Geometry check sheet. Reference: the model listing, model coordinates, mm. A direction names the side the tool comes from. Round coordinates to 2 decimals unless told otherwise and drop trailing zeros. Write each loop counter-clockwise with the first axis right and the second up, starting at its lowest first coordinate (ties: lowest second). Pieces come first, ordered by that corner, then holes. Notation, with made-up numbers: (27.5, 21.5) -> (84.5, 21.5) arc R24 ccw to (84.5, 57.5) -> close; hole circle Ø2 at (86, 55). An arc over 180 degrees is marked (long way). One line per question, with ' | ' between items.
```python
from build123d import *

# Parameters (mm, degrees)
ESQUISSE1_W                = 50
ESQUISSE1_H                = 10
BOSS_EXTRU_1_DEPTH         = 100
ESQUISSE2_R                = 5
BOSS_EXTRU_2_DEPTH         = 15
ESQUISSE3_R                = 5
BOSS_EXTRU_3_DEPTH         = 15
ESQUISSE4_W                = 10
ESQUISSE4_H                = 10
ENL_V_MAT_EXTRU_1_DEPTH    = 15
R_P_TITION_LIN_AIRE1_COUNT = 5
R_P_TITION_LIN_AIRE1_PITCH = 20
ESQUISSE5_W                = 10
ESQUISSE5_H                = 100
BOSS_EXTRU_4_DEPTH         = 40


with BuildPart() as part:
    # Esquisse1 → Boss.-Extru.1 (new body)
    with BuildSketch(Plane.XY):
        with Locations((-25, 5)):
            Rectangle(ESQUISSE1_W, ESQUISSE1_H)
    extrude(amount=BOSS_EXTRU_1_DEPTH)

    # Esquisse2 → Boss.-Extru.2 (add)
    with BuildSketch(Plane.XY.offset(100)):
        with Locations((-5, 5)):
            Circle(ESQUISSE2_R)
    extrude(amount=BOSS_EXTRU_2_DEPTH)

    # Esquisse3 → Boss.-Extru.3 (add)
    with BuildSketch(Plane(origin=(0, 0, 0), x_dir=(-1, 0, 0), z_dir=(0, 0, -1))):
        with Locations((5, 5)):
            Circle(ESQUISSE3_R)
    extrude(amount=BOSS_EXTRU_3_DEPTH)

    # Esquisse4 → Enlèv. mat.-Extru.1 (cut)
    with BuildSketch(Plane(origin=(0, 10, 0), x_dir=(1, 0, 0), z_dir=(0, 1, 0))):
        with Locations((-45, -5)):
            Rectangle(ESQUISSE4_W, ESQUISSE4_H)
    enl_v_mat_extru_1 = extrude(amount=-ENL_V_MAT_EXTRU_1_DEPTH, mode=Mode.SUBTRACT)

    # Répétition linéaire1: Enlèv. mat.-Extru.1 ×5
    with Locations(*[(0, 0, i * R_P_TITION_LIN_AIRE1_PITCH) for i in range(1, R_P_TITION_LIN_AIRE1_COUNT)]):
        add(enl_v_mat_extru_1, mode=Mode.SUBTRACT)

    # Esquisse5 → Boss.-Extru.4 (add)
    with BuildSketch(Plane(origin=(0, 10, 0), x_dir=(1, 0, 0), z_dir=(0, 1, 0))):
        with Locations((-5, -50)):
            Rectangle(ESQUISSE5_W, ESQUISSE5_H)
    extrude(amount=BOSS_EXTRU_4_DEPTH)


solid = part.part
```
(1) Go/stop test with flat-tipped pins: pin 1 (8 mm diameter, centred on x = -45, y = 4, fed in from -Z); pin 2 (4 mm diameter, centred on x = -25, z = 25.5, fed in from +Y); pin 3 (12 mm diameter, centred on y = 19, z = 24.5, fed in from -X). Record where each tip stops, or that it passes through.
Resolved:
pin 1: stops at z = 10 | pin 2: stops at y = 10 | pin 3: stops at x = -10
(2) Draft check along Z on faces 1 (the flat face through (-45, 5, 70)), 2 (the flat face through (-40, 5, 45)), 3 (the flat face through (-5, 5, -15)), 4 (the flat face through (-50, 5, 95)). Enter one of: +Z half, -Z half, draft (parallel to the pull), parting line (faces both ways), or undercut.
Resolved:
face 1: undercut | face 2: undercut | face 3: -Z half | face 4: draft
(3) Material ranges on line 1 (Z direction, x = -42, y = 7.5); line 2 (X direction, y = 47, z = 44); line 3 (Z direction, x = -6.5, y = 14), recorded low to high.
Resolved:
line 1: z = 10 to 20, 30 to 40, 50 to 60, 70 to 80, 90 to 100 | line 2: x = -10 to 0 | line 3: z = 0 to 100
(4) Sectioned sample at B-B on x = -8.5. Record the cut outline in (y, z), then the cut area to 3 significant figures.
Resolved:
outline: (0, 0) -> (1.43, 0) -> (1.43, -15) -> (8.57, -15) -> (8.57, 0) -> (50, 0) -> (50, 100) -> (8.57, 100) -> (8.57, 115) -> (1.43, 115) -> (1.43, 100) -> (0, 100) -> close | area: 5,210 mm2
(5) Sectioned sample at A-A on z = 6.5. Record the cut outline in (x, y).
Resolved:
outline: (-40, 0) -> (0, 0) -> (0, 50) -> (-10, 50) -> (-10, 10) -> (-40, 10) -> close
(6) Sectioned sample at D-D on x = -22. Record the cut outline in (y, z), then the cut area to 3 significant figures.
Resolved:
outline: (0, 0) -> (10, 0) -> (10, 100) -> (0, 100) -> close | area: 1,000 mm2
(7) Sectioned sample at C-C on y = 24. Record the cut outline in (x, z).
Resolved:
outline: (-10, 0) -> (0, 0) -> (0, 100) -> (-10, 100) -> close
(8) Access from +Z, -Z, +X, -X, +Y, -Y to the whole of each face (thin tool, end or side, straight path). Record for faces 5 (the flat face through (-45, 5, 90)), 6 (the flat face through (-30, 10, 49)), 7 (the cylindrical face through (-6.08, 0.12, 107.4)).
Resolved:
face 5: -X, +Y, -Y | face 6: +Z, -Z, -X, +Y | face 7: +Z
